Input: dimensioned drawing with shaded views. Units: mm. Origin: part minimum x, y, z. A direction names the side the tool comes from. Round coordinates to 2 decimals unless told otherwise and drop trailing zeros. Loops run counter-clockwise (first coordinate to the right, second up) from the corner with the lowest first, then second, coordinate; pieces in that order, holes last. Notation, with made-up numbers: M 10,62.25 L 30,62.25 A25 cw 30,76.25 Z; hole C -3.5,28 d11. An arc over 180 degrees is marked long. One line per item, written item: value.
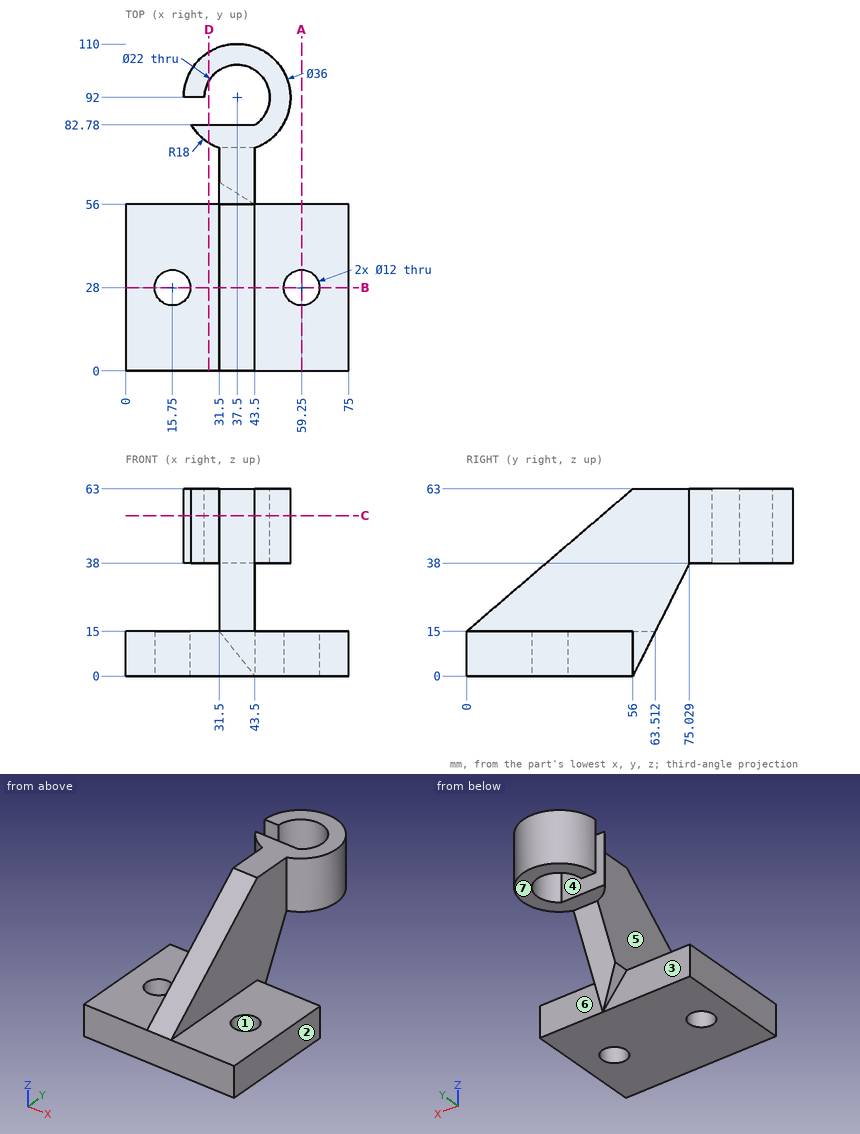
1. Section query C-C (z = 54). Return the cut outline in (x, y).
Report:
outline: M 19.5,92 L 26.5,92 A11 cw long 43.5,82.78 L 22.04,82.78 A18 ccw 31.5,75.03 L 31.5,45.5 L 43.5,45.5 L 43.5,75.03 A18 ccw long Z
2. Section query A-A (x = 59.25). Return the cut outline in (y, z).
Report:
outline: M 0,0 L 22,0 L 22,15 L 0,15 Z; M 34,0 L 56,0 L 56,15 L 34,15 Z
3. Pin query (flat end, axial travel): pin 1 (5 mm diameter, centred on y = 32, z = 40, fed in from +X); pin 2 (5.5 mm diameter, centred on x = 23, z = 52, fed in from -Y) (1 decimal); pin 3 (7.5 mm diameter, centred on x = 62, z = 7.5, fed in from +Y). Return the tip coordinate at first contact, or that it passes through.
Report:
pin 1: stops at x = 43.5
pin 2: stops at y = 78.4
pin 3: stops at y = 56
4. Ray query, line 1 (X direction, y = 28, z = 9); line 2 (Y direction, x = 15.75, z = 7.75); line 3 (X direction, y = 30, z = 27.5). Return the intervals inside material, ascending. Write a range as [from, to].
Report:
line 1: x = [0, 9.75], [21.75, 53.25], [65.25, 75]
line 2: y = [0, 22], [34, 56]
line 3: x = [31.5, 43.5]
5. Pull-direction query (Y, two-part tool) for the marked faces 1, 2, 3 and 4; classes: released by +Y, released by -Y, zero draft, split by the parting line, or undercut.
Report:
face 1: undercut
face 2: zero draft
face 3: released by +Y
face 4: undercut
6. Section query D-D (x = 28). Return the cut outline in (y, z) (1 decimal).
Report:
outline: M 0,0 L 56,0 L 56,15 L 0,15 Z; M 76.7,38 L 82.8,38 L 82.8,63 L 76.7,63 Z; M 97.5,38 L 107.3,38 L 107.3,63 L 97.5,63 Z
7. Section query B-B (y = 28). Return the cut outline in (x, z).
Report:
outline: M 0,0 L 9.75,0 L 9.75,15 L 0,15 Z; M 21.75,0 L 53.25,0 L 53.25,15 L 43.5,15 L 43.5,39 L 31.5,39 L 31.5,15 L 21.75,15 Z; M 65.25,0 L 75,0 L 75,15 L 65.25,15 Z
8. Reachability of the marked faces 5, 6 and 7 from +Z, -Z, +X, -X, +Y, -Y: full face, straight path, thin tool, end or side. Return the list, or none.
Report:
face 5: +Z, -X, -Y
face 6: +Z, -Z, +X, +Y
face 7: -Z, +X, -X, +Y
